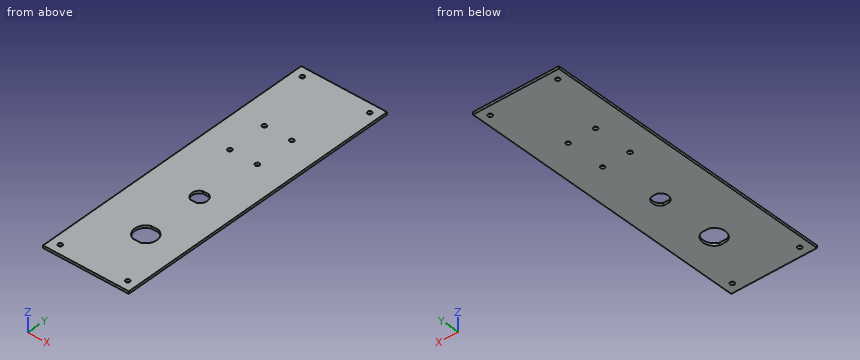
Autodesk Fusion 360 part; units mm, degrees
sketch "Sketch1" plane through (0, 0, 0) normal (0, 0, 1) x (1, 0, 0)
  line L0 (0, 0) -> (70, 0)
  line L1 (70, 0) -> (70, 240)
  line L2 (70, 240) -> (0, 240)
  line L3 (0, 240) -> (0, 0)
  dimension "d1" = 240
  dimension "d2" = 70
extrude "Extrude1" add sketch "Sketch1" along normal blind 2
sketch "Sketch2" plane through (0, 0, 2) normal (0, 0, 1) x (1, 0, 0)
  line L0 (0, 240) -> (0, 0)
  line L1 (0, 0) -> (70, 0)
  line L2 (70, 0) -> (70, 240)
  line L3 (70, 240) -> (0, 240)
  circle A0 centre (40, 50) radius 9
  line L4 (42.958, 41.5) -> (37.042, 41.5)
  line L5 (37.042, 41.5) -> (37.042, 58.5)
  line L6 (37.042, 58.5) -> (42.958, 58.5)
  line L7 (42.958, 58.5) -> (42.958, 41.5)
  circle A1 centre (40, 100) radius 6.25
  line L8 (42.4495, 94.25) -> (37.5505, 94.25)
  line L9 (37.5505, 94.25) -> (37.5505, 105.75)
  line L10 (37.5505, 105.75) -> (42.4495, 105.75)
  line L11 (42.4495, 105.75) -> (42.4495, 94.25)
  point P0 (35, 0)
  point P1 (40, 41.5)
  dimension "d5" = 18
  dimension "d6" = 17
  dimension "d7" = 50
  dimension "d8" = 12.5
  dimension "d9" = 11.5
  dimension "d10" = 50
  dimension "d14" = 40
extrude "Extrude2" cut sketch "Sketch2" against normal blind 15 contours A0 L7 | L4 L5 L6 L7 | A0 L5 | A1 L11 | L8 L9 L10 L11 | A1 L9
sketch "Sketch3" plane through (0, 0, 2) normal (0, 0, 1) x (1, 0, 0)
  line L0 (42.958, 41.5) -> (37.042, 41.5)
  arc A0 (37.042, 58.5) -> (37.042, 41.5) centre (40, 50) ccw
  line L1 (37.042, 58.5) -> (42.958, 58.5)
  arc A1 (42.958, 41.5) -> (42.958, 58.5) centre (40, 50) ccw
  line L2 (42.4495, 94.25) -> (37.5505, 94.25)
  arc A2 (37.5505, 105.75) -> (37.5505, 94.25) centre (40, 100) ccw
  line L3 (37.5505, 105.75) -> (42.4495, 105.75)
  arc A3 (42.4495, 94.25) -> (42.4495, 105.75) centre (40, 100) ccw
  line L4 (0, 240) -> (0, 0)
  line L5 (0, 0) -> (70, 0)
  line L6 (70, 0) -> (70, 240)
  line L7 (70, 240) -> (0, 240)
  circle A4 centre (7.5, 232.5) radius 1.75
  circle A5 centre (62.5, 232.5) radius 1.75
  circle A6 centre (62.5, 7.5) radius 1.75
  circle A7 centre (7.5, 7.5) radius 1.75
  line L8 (7.5, 232.5) -> (7.5, 7.5) construction
  line L9 (7.5, 7.5) -> (62.5, 7.5) construction
  line L10 (62.5, 7.5) -> (62.5, 232.5) construction
  line L11 (62.5, 232.5) -> (7.5, 232.5) construction
  dimension "d15" = 7.5
  dimension "d16" = 3.5
  dimension "d17" = 3.5
  dimension "d18" = 3.5
  dimension "d19" = 3.5
extrude "Extrude3" cut sketch "Sketch3" against normal blind 5 contours A4 | A5 | A6 | A7
sketch "Sketch4" plane through (0, 0, 2) normal (0, 0, 1) x (1, 0, 0)
  circle A0 centre (62.5, 232.5) radius 1.75
  circle A1 centre (7.5, 7.5) radius 1.75
  circle A2 centre (7.5, 232.5) radius 1.75
  circle A3 centre (62.5, 7.5) radius 1.75
  line L0 (42.958, 41.5) -> (37.042, 41.5)
  arc A4 (37.042, 58.5) -> (37.042, 41.5) centre (40, 50) ccw
  line L1 (37.042, 58.5) -> (42.958, 58.5)
  arc A5 (42.958, 41.5) -> (42.958, 58.5) centre (40, 50) ccw
  line L2 (42.4495, 94.25) -> (37.5505, 94.25)
  arc A6 (37.5505, 105.75) -> (37.5505, 94.25) centre (40, 100) ccw
  line L3 (37.5505, 105.75) -> (42.4495, 105.75)
  arc A7 (42.4495, 94.25) -> (42.4495, 105.75) centre (40, 100) ccw
  line L4 (0, 240) -> (0, 0)
  line L5 (0, 0) -> (70, 0)
  line L6 (70, 0) -> (70, 240)
  line L7 (70, 240) -> (0, 240)
  circle A8 centre (22.648, 147.996) radius 1.75
  circle A9 centre (22.648, 180) radius 1.75
  circle A10 centre (45, 147.996) radius 1.75
  circle A11 centre (45, 180) radius 1.75
  dimension "d22" = 3.5
  dimension "d23" = 3.5
  dimension "d24" = 32.004
  dimension "d25" = 3.5
  dimension "d26" = 3.5
  dimension "d27" = 22.352
  dimension "d28" = 25
  dimension "d29" = 60
extrude "Extrude4" cut sketch "Sketch4" against normal blind 5 contours A8 | A9 | A10 | A11
equation "d1 = 210 mm + 30 mm"
equation "d17 = d16"
equation "d18 = d16"
equation "d19 = d16"
equation "d23 = d22"
equation "d25 = d22"
equation "d26 = d23"
equation "d27 = 1 in - 0.12 in"
The model under review builds one solid part; all positions refer to its coordinate system, in mm. Coordinates: 2 decimals unless noted, no trailing zeros.
(1) Insertion check: P1, Ø2, axis at x = 22.648, y = 180, coming from the -Z side. The pin has a flat end and moves straight along its axis. Give the tip position at first contact, or say it passes through.
Determined:
P1: passes through
(2) Consider section A-A, the plane z = 1.7. Give the number of separate pieces and of enclosed holes in the cut face, plus the area to 3 significant figures.
Determined:
separate pieces: 1
enclosed holes: 10
area: 16,400 mm2
(3) Wall thickness on L1, parallel to X at y = 232.5, z = 1.1; L2, parallel to Y at x = 7.5, z = 1.4; L3, parallel to X at y = 180, z = 1.5: over which ranges is each line inside the solid? List them lowest first.
Determined:
L1: x = 0 to 5.75, 9.25 to 60.75, 64.25 to 70
L2: y = 0 to 5.75, 9.25 to 230.75, 234.25 to 240
L3: x = 0 to 20.9, 24.4 to 43.25, 46.75 to 70
